```python
from build123d import *

# Parameters (mm, degrees)
SKETCH1_R           = 12.7
SKETCH1_R_2         = 4.7625
SKETCH1_W           = 3.175
SKETCH1_H           = 50.8
BOSS_EXTRUDE1_DEPTH = 7.62
CUT_EXTRUDE1_DEPTH  = 7.62


with BuildPart() as part:
    # Sketch1 → Boss-Extrude1 (new body)
    # profile 1 of 2: a face of its own
    with BuildSketch(Plane.XY):
        with Locations((-11.43, -2.615954226)):
            Circle(SKETCH1_R)
        with Locations((-11.43, -2.615954226)):
            Circle(SKETCH1_R_2, mode=Mode.SUBTRACT)
    # profile 2 of 2: a face of its own
    with BuildSketch(Plane.XY):
        with Locations((1.5875, -2.615954226)):
            Rectangle(SKETCH1_W, SKETCH1_H)
    extrude(amount=BOSS_EXTRUDE1_DEPTH)

    # Sketch3 → Cut-Extrude1 (cut)
    with BuildSketch(Plane(origin=(5.715, 0, 0), x_dir=(0, 0, -1), z_dir=(1, 0, 0))):
        with BuildLine():
            ThreePointArc((-0.81, 15.116671426), (-1.688679656, 17.237991769), (-3.81, 18.116671426))
            Line((-3.81, 18.116671426), (-3.81, 15.116671426))
            Line((-3.81, 15.116671426), (-3.81, 12.116671426))
            ThreePointArc((-3.81, 12.116671426), (-1.688679656, 12.995351082), (-0.81, 15.116671426))
        make_face()
        with BuildLine():
            Line((-3.81, 15.116671426), (-3.81, 18.116671426))
            ThreePointArc((-3.81, 18.116671426), (-6.81, 15.116671426), (-3.81, 12.116671426))
            Line((-3.81, 12.116671426), (-3.81, 15.116671426))
        make_face()
        with BuildLine():
            ThreePointArc((-0.81, -20.395954226), (-1.688679656, -18.274633882), (-3.81, -17.395954226))
            Line((-3.81, -17.395954226), (-3.81, -20.395954226))
            Line((-3.81, -20.395954226), (-3.81, -23.395954226))
            ThreePointArc((-3.81, -23.395954226), (-1.688679656, -22.517274569), (-0.81, -20.395954226))
        make_face()
        with BuildLine():
            Line((-3.81, -20.395954226), (-3.81, -17.395954226))
            ThreePointArc((-3.81, -17.395954226), (-6.81, -20.395954226), (-3.81, -23.395954226))
            Line((-3.81, -23.395954226), (-3.81, -20.395954226))
        make_face()
    extrude(amount=-CUT_EXTRUDE1_DEPTH, mode=Mode.SUBTRACT)


solid = part.part
```
Can you work these out from the model? Positions are in its coordinate system, mm. A direction names the side the tool comes from. Coordinates: 2 decimals unless noted, no trailing zeros. Loops run counter-clockwise (first coordinate to the right, second up) from the corner with the lowest first, then second, coordinate; pieces in that order, holes last. Notation, with made-up numbers: (76.25, 56.25) -> (122.25, 56.25) arc R31 cw to (122.25, 82.25) -> close; hole circle Ø7 at (29.5, 88). An arc over 180 degrees is marked (long way). Put each result on its own line as item: value. Start each with the question number.
Q1. I want a section at A-A (z = 2.75). Write out the boundary of the cut face in (x, y) (1 decimal), plus the area to 3 significant figures.
Q2. I want a section at B-B (y = 7.5). Write out the boundary of the cut face in (x, z) (3 decimals), plus the area to 3 significant figures.
Q3. Thinking about a two-plate mould opening in X: for faces 4 (the face through (2, -28.016, 4)), 5 (the face through (3.175, -3, 4)), 6 (the face through (-24.12, -2.14, 3.76)), which applies, pulls with the +X half, pulls with the -X half, needs draft (parallel to the pull), parting line crosses it, or undercut?
Q4. I'm going to push flat-ended pins straight in: P1, Ø11, axis at x = -11.43, y = -2.62, coming from the +Z side; P2, Ø4, axis at y = 12.5, z = 2, coming from the -X side; P3, Ø2, axis at x = -20.5, z = 5.5, coming from the +Y side; P4, Ø12, axis at x = -18.5, y = 15.5, coming from the -Z side. Where does each tip first touch, or does it pass through?
Q5. For faces 1 (the face through (-5, -2, 0)), 2 (the face through (0, -16, 4)), 3 (the face through (0, 11, 4)), which set-ups out of +Z, -Z, +X, -X, +Y, -Y let a thin tool reach every point of the face, with its end or its side?
Q6. If I drill on line 1 (X direction, y = -2.5, z = 2.75) (3 decimals); line 2 (Y direction, x = -11.43, z = 4.75); line 3 (Z direction, x = 0.5, y = 15), over which ranges is the centre line in solid material (lowest first)? Write a range as [from, to].
Q7. I want a section at C-C (x = -11.75). Write out the boundary of the cut face in (y, z), plus the area to 3 significant figures.
Q8. I want a section at D-D (z = 5.5). Write out the boundary of the cut face in (x, y) (1 decimal), plus the area to 3 significant figures.
Taken from the geometry:
1. outline: (0, -28) -> (3.2, -28) -> (3.2, -23.2) -> (0, -23.2) -> close; (0, -17.6) -> (3.2, -17.6) -> (3.2, 12.3) -> (0, 12.3) -> (0, 2.9) arc R12.7 ccw (long way) to (0, -8.2) -> close; (0, 17.9) -> (3.2, 17.9) -> (3.2, 22.8) -> (0, 22.8) -> close; hole circle Ø9.5 at (-11.4, -2.6)
1. area: 552 mm2
2. outline: (-19.108, 0) -> (-3.752, 0) -> (-3.752, 7.62) -> (-19.108, 7.62) -> close; (0, 0) -> (3.175, 0) -> (3.175, 7.62) -> (0, 7.62) -> close
2. area: 141 mm2
3. face 4: needs draft
3. face 5: pulls with the +X half
3. face 6: undercut
4. P1: stops at z = 7.62
4. P2: stops at x = 0
4. P3: stops at y = 7.19
4. P4: passes through
5. face 1: -Z, +X, -X, +Y, -Y
5. face 2: +Z, -Z, -Y
5. face 3: +Z, -Z, +Y
6. line 1: x = [-24.129, -16.191], [-6.669, 3.175]
6. line 2: y = [-15.32, -7.38], [2.15, 10.08]
6. line 3: z = [0, 0.81], [6.81, 7.62]
7. outline: (-15.31, 0) -> (-7.37, 0) -> (-7.37, 7.62) -> (-15.31, 7.62) -> close; (2.14, 0) -> (10.08, 0) -> (10.08, 7.62) -> (2.14, 7.62) -> close
7. area: 121 mm2
8. outline: (0, -28) -> (3.2, -28) -> (3.2, -22.9) -> (0, -22.9) -> close; (0, -17.9) -> (3.2, -17.9) -> (3.2, 12.6) -> (0, 12.6) -> (0, 2.9) arc R12.7 ccw (long way) to (0, -8.2) -> close; (0, 17.6) -> (3.2, 17.6) -> (3.2, 22.8) -> (0, 22.8) -> close; hole circle Ø9.5 at (-11.4, -2.6)
8. area: 556 mm2
